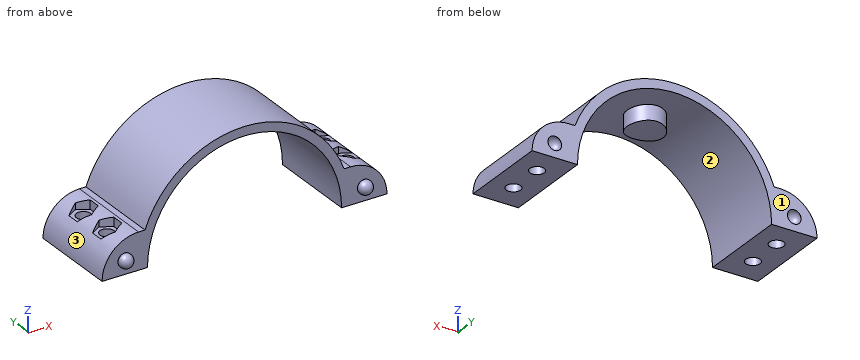
```python
from build123d import *

# Parameters (mm, degrees)
BOSS_EXTRUDE5_DEPTH      = 12.7
BOSS_EXTRUDE5_DEPTH_BACK = 12.7
SKETCH6_R                = 2.000000064
CUT_EXTRUDE4_DEPTH       = 52.101224931
CUT_EXTRUDE5_START       = -7.62
CUT_EXTRUDE5_DEPTH       = 2.54
SKETCH9_R                = 1.905
BOSS_EXTRUDE9_DEPTH      = 0.0254
DOME3_FACE_RADIUS        = 1.905
DOME3_HEIGHT             = 2.286
DOME4_FACE_RADIUS        = 1.905
DOME4_HEIGHT             = 2.286
SKETCH10_R               = 1.905
CUT_EXTRUDE6_DEPTH       = 0.0254
DOME5_FACE_RADIUS        = 1.905
DOME5_HEIGHT             = 2.286
DOME6_FACE_RADIUS        = 1.905
DOME6_HEIGHT             = 2.286
BOSS_EXTRUDE10_START     = -28
BOSS_EXTRUDE10_DEPTH     = 9.812276711
BOSS_EXTRUDE10_START_2   = -6
BOSS_EXTRUDE10_2_DEPTH   = 12
CUT_EXTRUDE7_DEPTH       = 10.414
CUT_EXTRUDE7_DEPTH_BACK  = 10.414
SKETCH13_R               = 22.86


with BuildPart() as part:
    # Sketch3 → Boss-Extrude5 (new, two sides: drawn at the far end of the back side and taken through both)
    with BuildSketch(Plane(origin=(0, 0, 0), x_dir=(-1, 0, 0), z_dir=(0, -1, 0)).offset(-BOSS_EXTRUDE5_DEPTH_BACK)):
        with BuildLine():
            Line((27.051, 0), (29.549701049, 0))
            Line((29.549701049, 0), (39.709701049, 0))
            ThreePointArc((39.709701049, 0), (36.733905946, -7.184204897), (29.549701049, -10.16))
            Line((29.549701049, -10.16), (27.748139255, -10.16))
            ThreePointArc((27.748139255, -10.16), (0, -29.549701049), (-27.748139255, -10.16))
            Line((-27.748139255, -10.16), (-29.549701049, -10.16))
            ThreePointArc((-29.549701049, -10.16), (-36.733905946, -7.184204897), (-39.709701049, 0))
            Line((-39.709701049, 0), (-29.549701049, 0))
            Line((-29.549701049, 0), (-27.051, 0))
            ThreePointArc((-27.051, 0), (0, -27.051), (27.051, 0))
        make_face()
    extrude(amount=BOSS_EXTRUDE5_DEPTH + BOSS_EXTRUDE5_DEPTH_BACK)

    # Sketch6 → Cut-Extrude4 (cut, through all)
    with BuildSketch(Plane(origin=(0, 0, 0), x_dir=(-1, 0, 0), z_dir=(0, 0, -1))):
        with Locations((-33.380350525, 5.08)):
            Circle(SKETCH6_R)
        with Locations((-33.380350525, -5.08)):
            Circle(SKETCH6_R)
        with Locations((33.380350525, 5.08)):
            Circle(SKETCH6_R)
        with Locations((33.380350525, -5.08)):
            Circle(SKETCH6_R)
    extrude(amount=-CUT_EXTRUDE4_DEPTH, mode=Mode.SUBTRACT)

    # Sketch7 → Cut-Extrude5 (cut)
    with BuildSketch(Plane(origin=(0, 0, 0), x_dir=(-1, 0, 0), z_dir=(0, 0, -1)).offset(CUT_EXTRUDE5_START)):
        Polygon((-30.380350525, 6.812050808), (-33.380350525, 8.544101615), (-36.380350525, 6.812050808), (-36.380350525, 3.347949192), (-33.380350525, 1.615898385), (-30.380350525, 3.347949192), align=None)
        Polygon((-30.380350525, -3.347949192), (-33.380350525, -1.615898385), (-36.380350525, -3.347949192), (-36.380350525, -6.812050808), (-33.380350525, -8.544101615), (-30.380350525, -6.812050808), align=None)
        Polygon((36.380350525, 6.812050808), (33.380350525, 8.544101615), (30.380350525, 6.812050808), (30.380350525, 3.347949192), (33.380350525, 1.615898385), (36.380350525, 3.347949192), align=None)
        Polygon((36.380350525, -3.347949192), (33.380350525, -1.615898385), (30.380350525, -3.347949192), (30.380350525, -6.812050808), (33.380350525, -8.544101615), (36.380350525, -6.812050808), align=None)
    extrude(amount=-CUT_EXTRUDE5_DEPTH, mode=Mode.SUBTRACT)

    # Sketch9 → Boss-Extrude9 (add)
    with BuildSketch(Plane(origin=(0, -12.7, 0), x_dir=(-1, 0, 0), z_dir=(0, -1, 0))):
        with Locations(Location((-33.380350525, -3.81, 0), (0, 0, 90))):
            Circle(SKETCH9_R)
        with Locations(Location((33.380350525, -3.81, 0), (0, 0, 90))):
            Circle(SKETCH9_R)
    extrude(amount=BOSS_EXTRUDE9_DEPTH)

    # Dome3: a dome of height H over a round flat face of radius A is a cap of a sphere of radius (A * A + H * H) / (2 * H)
    dome3_r = (DOME3_FACE_RADIUS * DOME3_FACE_RADIUS + DOME3_HEIGHT * DOME3_HEIGHT) / (2 * DOME3_HEIGHT)
    dome3_base = Plane((33.380350525, -12.7254, 3.81), z_dir=(0, -1, 0))
    with Locations(dome3_base.offset(DOME3_HEIGHT - dome3_r)):
        dome3_ball = Sphere(dome3_r, mode=Mode.PRIVATE)
    add(split(dome3_ball, bisect_by=dome3_base, keep=Keep.TOP, mode=Mode.PRIVATE))

    # Dome4: a dome of height H over a round flat face of radius A is a cap of a sphere of radius (A * A + H * H) / (2 * H)
    dome4_r = (DOME4_FACE_RADIUS * DOME4_FACE_RADIUS + DOME4_HEIGHT * DOME4_HEIGHT) / (2 * DOME4_HEIGHT)
    dome4_base = Plane((-33.380350525, -12.7254, 3.81), z_dir=(0, -1, 0))
    with Locations(dome4_base.offset(DOME4_HEIGHT - dome4_r)):
        dome4_ball = Sphere(dome4_r, mode=Mode.PRIVATE)
    add(split(dome4_ball, bisect_by=dome4_base, keep=Keep.TOP, mode=Mode.PRIVATE))

    # Sketch10 → Cut-Extrude6 (cut)
    with BuildSketch(Plane(origin=(0, 12.7, 0), x_dir=(1, 0, 0), z_dir=(0, 1, 0))):
        with Locations(Location((33.380350525, -3.81, 0), (0, 0, 90))):
            Circle(SKETCH10_R)
        with Locations(Location((-33.380350525, -3.81, 0), (0, 0, 90))):
            Circle(SKETCH10_R)
    extrude(amount=-CUT_EXTRUDE6_DEPTH, mode=Mode.SUBTRACT)

    # Dome5: a dome of height H over a round flat face of radius A is a cap of a sphere of radius (A * A + H * H) / (2 * H)
    dome5_r = (DOME5_FACE_RADIUS * DOME5_FACE_RADIUS + DOME5_HEIGHT * DOME5_HEIGHT) / (2 * DOME5_HEIGHT)
    dome5_base = Plane((33.380350525, 12.6746, 3.81), z_dir=(0, -1, 0))
    with Locations(dome5_base.offset(DOME5_HEIGHT - dome5_r)):
        dome5_ball = Sphere(dome5_r, mode=Mode.PRIVATE)
    add(split(dome5_ball, bisect_by=dome5_base, keep=Keep.TOP, mode=Mode.PRIVATE), mode=Mode.SUBTRACT)

    # Dome6: a dome of height H over a round flat face of radius A is a cap of a sphere of radius (A * A + H * H) / (2 * H)
    dome6_r = (DOME6_FACE_RADIUS * DOME6_FACE_RADIUS + DOME6_HEIGHT * DOME6_HEIGHT) / (2 * DOME6_HEIGHT)
    dome6_base = Plane((-33.380350525, 12.6746, 3.81), z_dir=(0, -1, 0))
    with Locations(dome6_base.offset(DOME6_HEIGHT - dome6_r)):
        dome6_ball = Sphere(dome6_r, mode=Mode.PRIVATE)
    add(split(dome6_ball, bisect_by=dome6_base, keep=Keep.TOP, mode=Mode.PRIVATE), mode=Mode.SUBTRACT)

    # Boss-Extrude10: read off the stored shape, not the designer's step
    # Boss-Extrude10 outline → Boss-Extrude10 (add)
    with BuildSketch(Plane(origin=(0, 0, 0), x_dir=(-1, 0, 0), z_dir=(0, 0, -1)).offset(BOSS_EXTRUDE10_START)):
        with BuildLine():
            add(Edge.make_bspline(
                [(5.08, 0), (5.08, -1.345643562), (4.526719274, -2.65770318), (2.656649507, -4.527337736), (1.331455476, -5.079221738), (-1.32551012, -5.080776522), (-2.646103693, -4.537670622), (-4.536464951, -2.648170155), (-5.07946682, -1.329666265), (-5.080532362, 1.325589104), (-4.531084206, 2.651405113), (-2.659686169, 4.526228301), (-1.345855952, 5.079004988), (1.338333997, 5.080992228), (2.654502959, 4.528337308), (4.524460769, 2.661104937), (5.08, 1.345643562), (5.08, 0)],
                knots=[0, 0, 0, 0, 0.125, 0.125, 0.25, 0.25, 0.375, 0.375, 0.5, 0.5, 0.625, 0.625, 0.75, 0.75, 0.875, 0.875, 1, 1, 1, 1], degree=3))
        make_face()
    extrude(amount=BOSS_EXTRUDE10_DEPTH)

    # Boss-Extrude10 2 outline → Boss-Extrude10 2 (cut)
    with BuildSketch(Plane(origin=(0, 0, 0), x_dir=(1, 0, 0), z_dir=(0, 1, 0)).offset(BOSS_EXTRUDE10_START_2)):
        with BuildLine():
            Line((5.080000094, -18.187723372), (-5.080000481, -18.187723298))
            ThreePointArc((-5.080000481, -18.187723298), (-1.97e-07, -18.669), (5.080000094, -18.187723372))
        make_face()
    extrude(amount=BOSS_EXTRUDE10_2_DEPTH, mode=Mode.SUBTRACT)

    # Sketch13 → Cut-Extrude7 (cut, two sides: drawn at the far end of the back side and taken through both)
    with BuildSketch(Plane(origin=(0, 0, 0), x_dir=(1, 0, 0), z_dir=(0, 1, 0)).offset(-CUT_EXTRUDE7_DEPTH_BACK)):
        Circle(SKETCH13_R)
    extrude(amount=CUT_EXTRUDE7_DEPTH + CUT_EXTRUDE7_DEPTH_BACK, mode=Mode.SUBTRACT)


solid = part.part
```
Model file for the job. Use its own axes, mm. Face numbers are marked on the shaded views. Coordinates: 2 decimals unless noted, no trailing zeros. Loops run counter-clockwise (first coordinate to the right, second up) from the corner with the lowest first, then second, coordinate; pieces in that order, holes last. Notation, with made-up numbers: (49.5, 63) -> (82.5, 63) arc R15 ccw to (82.5, 77) -> close; hole circle Ø4 at (-16, 5.5). An arc over 180 degrees is marked (long way). Answer as a JSON object with one key per item and string values.
Q1. Cut at C-C (x = 18.5). List the corners of the cut face in (y, z).
Report:
{"outline": "(-12.7, 19.74) -> (12.7, 19.74) -> (12.7, 23.04) -> (-12.7, 23.04) -> close"}
Q2. Cut at A-A (z = 3.81). State how many separate pieces and enclosed holes the cut face has, and give its area (3 significant figures).
Report:
{"separate pieces": "2", "enclosed holes": "4", "area": "569 mm2"}
Q3. Cut at D-D (z = 21). List the corners of the cut face in (x, y), and give its area (3 significant figures).
Report:
{"outline": "(-20.79, -12.7) -> (-17.05, -12.7) -> (-17.05, 12.7) -> (-20.79, 12.7) -> close; (17.05, -12.7) -> (20.79, -12.7) -> (20.79, 12.7) -> (17.05, 12.7) -> close", "area": "190 mm2"}
Q4. Flat gauge pins, fed straight in: P1, Ø0.8, axis at y = 4.5, z = 9.5, coming from the -X side; P2, Ø4.5, axis at x = 32, y = -6.5, coming from the +Z side; P3, Ø3, axis at x = -33, y = -4, coming from the +Z side. Where does each tip first touch, or does it go through?
Report:
{"P1": "stops at x = -30.38", "P2": "stops at z = 10.16", "P3": "stops at z = 7.62"}
Q5. Pull direction X, two halves, no side cores. Call the marked faces 1, 2 and 3: released by +X, released by -X, zero draft, split by the parting line, or undercut.
Report:
{"face 1": "zero draft", "face 2": "undercut", "face 3": "released by -X"}
Q6. Probe probe 1 along X at (y, z) = (3.75, 7.5); probe 2 along Z at (x, y) = (29, 0.25); probe 3 along X at (y, z) = (-7.5, 14.5). List the from-to ranges inside material, lowest first.
Report:
{"probe 1": "x = -36.4 to -34.87, -31.89 to -25.99, 25.99 to 31.89, 34.87 to 36.4", "probe 2": "z = 0 to 10.16", "probe 3": "x = -25.75 to -22.84, 22.84 to 25.75"}
